Build history of the part. All positions in model axes, mm. A direction names the side the tool comes from. Round coordinates to 2 decimals unless told otherwise and drop trailing zeros. Write each loop counter-clockwise with the first axis right and the second up, starting at its lowest first coordinate (ties: lowest second). Pieces come first, ordered by that corner, then holes. Notation, with made-up numbers: M -30,42.5 L 29,42.5 A14 ccw 29,47.5 Z; hole C -30.75,89.25 d3. An arc over 180 degrees is marked long. Write item = value, one per line. Start each with the question number.
Q1. Band-saw the part on D-D on z = -16. Write the cut outline in (x, y), plus the area to 3 significant figures.
Q2. Probe L1, parallel to Z at x = -3.5, y = 17.5; L2, parallel to Y at x = 0, z = 1.2; L3, parallel to Z at x = 3, y = 15. List the from-to ranges inside material, lowest first.
Q3. Drop flat-ended pins along their axis: P1, Ø2, axis at x = -1.5, y = -0.5, coming from the +Z side; P2, Ø12, axis at y = 20.5, z = -8, coming from the +X side; P3, Ø3.5, axis at x = -0.5, y = -1.5, coming from the -Z side; P4, Ø1, axis at x = -1.5, z = -3, coming from the +Y side. Give the stop position or say it passes through.
Q4. Pull direction Y, two halves, no side cores. Call faces 1 (the cylindrical face through (2.1, 0.66, 0.04)), 2 (the cylindrical face through (-0.05, 5.07, 2.87)), 3 (the flat face through (-0.05, 14.54, -8.96)): released by +Y, released by -Y, zero draft, split by the parting line, or undercut.
Q5. Band-saw the part on B-B on y = 17. Write the cut outline in (x, z), plus the area to 3 significant figures.
Q6. Band-saw the part on A-A on x = 0. Write the cut outline in (y, z), plus the area to 3 significant figures.
Q7. Band-saw the part on C-C on z = -0.5. Write the cut outline in (x, y), plus the area to 3 significant figures.
Q8. Tool access for faces 4 (the flat face through (-2, -2, -2.5)), 5 (the flat face through (3, 0, 2.5)), 6 (the flat face through (-0.05, 14.79, 9.21)): list every direction of +Z, -Z, +X, -X, +Y, -Y with a clear straight run to the whole face (end or side of a thin tool).
```python
from build123d import *

# Parameters (mm, degrees)
BOSS_EXTRUDE1_DEPTH             = 2.5
BOSS_EXTRUDE2_REACH             = 7.863
BOSS_EXTRUDE2_DIRECTION_2_REACH = 7.863
CUT_EXTRUDE2_DEPTH              = 33.577791515
CUT_EXTRUDE2_DEPTH_BACK         = 33.577791515
SKETCH5_W                       = 5
SKETCH5_H                       = 1.5
BOSS_EXTRUDE3_DEPTH             = 7.5
SKETCH6_R                       = 2.2
CUT_EXTRUDE4_DEPTH              = 10
FILLET1_R                       = 5


with BuildPart() as part:
    # Sketch1 → Boss-Extrude1 (new, symmetric)
    with BuildSketch(Plane.XY):
        with BuildLine():
            Line((-3.75, 0), (-3.75, 3.75))
            Line((-3.75, 3.75), (3.75, 3.75))
            Line((3.75, 3.75), (3.75, 0))
            ThreePointArc((3.75, 0), (0, -3.75), (-3.75, 0))
        make_face()
    extrude(amount=BOSS_EXTRUDE1_DEPTH, both=True)

    # Boss-Extrude2: up to this face of the body (flat: up to its plane)
    boss_extrude2_end = Plane(part.part.faces().sort_by_distance((3.75, 1.875, 0))[0])
    # Sketch3 → Boss-Extrude2 (add, up to the picked face)
    with BuildSketch(Plane(origin=(0, 0, 0), x_dir=(0, 0, -1), z_dir=(1, 0, 0)), mode=Mode.PRIVATE) as boss_extrude2_sk1:
        Polygon((0, 2.75), (21, 23.75), (-21, 23.75), align=None)
    boss_extrude2_tool1 = split(extrude(boss_extrude2_sk1.sketch, amount=BOSS_EXTRUDE2_REACH, mode=Mode.PRIVATE), bisect_by=boss_extrude2_end, keep=Keep.BOTH, mode=Mode.PRIVATE)
    add(boss_extrude2_tool1.solids().sort_by(Axis((0, 16.75, 0), (1, 0, 0)))[0])

    # Boss-Extrude2 direction 2: up to this face of the body (flat: up to its plane)
    boss_extrude2_direction_2_end = Plane(part.part.faces().sort_by_distance((-3.75, 1.875, 0))[0])
    # Sketch3 → Boss-Extrude2 direction 2 (add, up to the picked face)
    with BuildSketch(Plane(origin=(0, 0, 0), x_dir=(0, 0, -1), z_dir=(1, 0, 0)), mode=Mode.PRIVATE) as boss_extrude2_direction_2_sk1:
        Polygon((0, 2.75), (21, 23.75), (-21, 23.75), align=None)
    boss_extrude2_direction_2_tool1 = split(extrude(boss_extrude2_direction_2_sk1.sketch, amount=-BOSS_EXTRUDE2_DIRECTION_2_REACH, mode=Mode.PRIVATE), bisect_by=boss_extrude2_direction_2_end, keep=Keep.BOTH, mode=Mode.PRIVATE)
    add(boss_extrude2_direction_2_tool1.solids().sort_by(Axis((0, 16.75, 0), (-1, 0, 0)))[0])

    # Sketch4 → Cut-Extrude2 (cut, two sides: drawn at the far end of the back side and taken through both)
    with BuildSketch(Plane(origin=(3.75, 0, 0), x_dir=(0, 0, -1), z_dir=(1, 0, 0)).offset(-CUT_EXTRUDE2_DEPTH_BACK)):
        Polygon((-18.171572875, 23.75), (0, 5.578427125), (18.171572875, 23.75), align=None)
    extrude(amount=CUT_EXTRUDE2_DEPTH + CUT_EXTRUDE2_DEPTH_BACK, mode=Mode.SUBTRACT)

    # Sketch5 → Boss-Extrude3 (add)
    with BuildSketch(Plane(origin=(3.75, 0, 0), x_dir=(0, 0, -1), z_dir=(1, 0, 0))):
        with Locations((0, 4.5)):
            Rectangle(SKETCH5_W, SKETCH5_H)
    extrude(amount=-BOSS_EXTRUDE3_DEPTH)

    # Sketch6 → Cut-Extrude4 (cut)
    with BuildSketch(Plane.XY.offset(2.5)):
        Circle(SKETCH6_R)
    extrude(amount=-CUT_EXTRUDE4_DEPTH, mode=Mode.SUBTRACT)

    # Fillet1
    fillet1_edges = [part.edges().sort_by_distance(p)[0] for p in [
        (0, 5.25, 2.5),
        (0, 5.25, -2.5),
    ]]
    fillet(fillet1_edges, radius=FILLET1_R)


solid = part.part
```
Conclusion:
q1.outline = M -3.75,18.75 L 3.75,18.75 L 3.75,21.58 L -3.75,21.58 Z
q1.area = 21.2 mm^2
q2.L1 = -14.75 to -11.92, 11.92 to 14.75
q2.L2 = -3.75 to -2.2, 2.2 to 6.78
q2.L3 = -12.25 to -9.42, 9.42 to 12.25
q3.P1 = 2.5
q3.P2 = 3.75
q3.P3 = -2.5
q3.P4 = 9.08
q4.face_1 = undercut
q4.face_2 = released by -Y
q4.face_3 = released by +Y
q5.outline = M -3.75,-14.25 L 3.75,-14.25 L 3.75,-11.42 L -3.75,-11.42 Z; M -3.75,11.42 L 3.75,11.42 L 3.75,14.25 L -3.75,14.25 Z
q5.area = 42.4 mm^2
q6.outline = M -3.75,-2.5 L -2.2,-2.5 L -2.2,2.5 L -3.75,2.5 Z; M 2.2,-2.5 L 3.18,-2.5 A5 cw 6.71,-3.96 L 23.75,-21 L 23.75,-18.17 L 5.58,0 L 23.75,18.17 L 23.75,21 L 6.71,3.96 A5 cw 3.18,2.5 L 2.2,2.5 Z
q6.area = 129 mm^2
q7.outline = M -3.75,0 A3.75 ccw 3.75,0 L 3.75,6.08 L -3.75,6.08 Z; hole C 0,0 d4.4
q7.area = 52.5 mm^2
q8.face_4 = -Z, +X, -X, -Y
q8.face_5 = +Z, +X, -X, -Y
q8.face_6 = +X, -X, +Y
